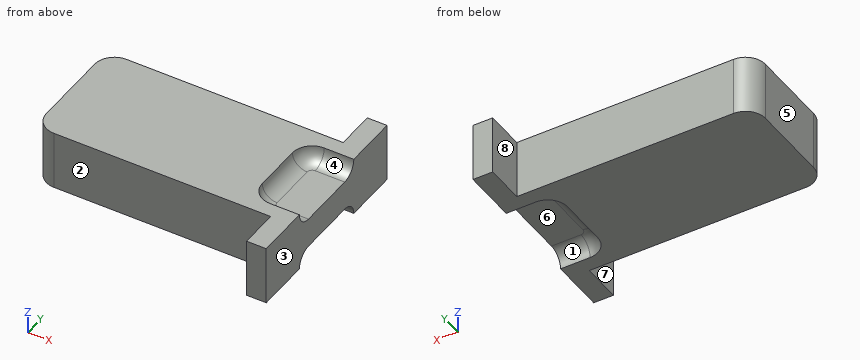
from build123d import *

# Parameters (mm, degrees)
F1_DEPTH = 9.525
F2_R     = 6.35
F4_DEPTH = 4.7625
F5_R     = 4.76249
F7_DEPTH = 4.7625
F8_R     = 4.76249


# Not quite as in the source:
# - a fillet or chamfer is up to 0.001 mm smaller than in the source, because OpenCascade refuses the exact size


with BuildPart() as f1:
    # F0 (on Top) → F1 (new body, symmetric)
    with BuildSketch(Plane.XY):
        Polygon((-82.55, 19.05), (-82.55, -19.05), (-6.35, -19.05), (-6.35, -31.75), (0, -31.75), (0, 31.75), (-6.35, 31.75), (-6.35, 19.05), align=None)
    extrude(amount=F1_DEPTH, both=True)

    # F2
    f2_edges = [f1.edges().sort_by_distance(p)[0] for p in [
        (-82.55, -19.05, 0),
        (-82.55, 19.05, 0),
    ]]
    fillet(f2_edges, radius=F2_R)

    # F3 (on face) → F4 (cut)
    with BuildSketch(Plane.XY.offset(9.525)):
        with BuildLine():
            Line((0, -14.2875), (0, 14.2875))
            Line((0, 14.2875), (-9.525, 14.2875))
            ThreePointArc((-9.525, 14.2875), (-14.0151280605, 12.4276280605), (-15.875, 7.9375))
            Line((-15.875, 7.9375), (-15.875, -7.9375))
            ThreePointArc((-15.875, -7.9375), (-14.0151280605, -12.4276280605), (-9.525, -14.2875))
            Line((-9.525, -14.2875), (0, -14.2875))
        make_face()
    extrude(amount=-F4_DEPTH, mode=Mode.SUBTRACT)

    # F5 (radius 4.7625 in the source; OpenCascade refuses exactly that, so slightly less here)
    f5_edges = [f1.edges().sort_by_distance(p)[0] for p in [
        (-4.7625, 14.2875, 4.7625),
        (-14.015128, 12.427628, 4.7625),
    ]]
    fillet(f5_edges, radius=F5_R)

    # F6 (on face) → F7 (cut)
    with BuildSketch(Plane(origin=(0, 0, -9.525), x_dir=(1, 0, 0), z_dir=(0, 0, -1))):
        with BuildLine():
            Line((0, -14.2875), (0, 14.2875))
            Line((0, 14.2875), (-9.525, 14.2875))
            ThreePointArc((-9.525, 14.2875), (-14.0151280605, 12.4276280605), (-15.875, 7.9375))
            Line((-15.875, 7.9375), (-15.875, -7.9375))
            ThreePointArc((-15.875, -7.9375), (-14.0151280605, -12.4276280605), (-9.525, -14.2875))
            Line((-9.525, -14.2875), (0, -14.2875))
        make_face()
    extrude(amount=-F7_DEPTH, mode=Mode.SUBTRACT)

    # F8 (radius 4.7625 in the source; OpenCascade refuses exactly that, so slightly less here)
    f8_edges = [f1.edges().sort_by_distance(p)[0] for p in [
        (-4.7625, -14.2875, -4.7625),
        (-14.015128, -12.427628, -4.7625),
    ]]
    fillet(f8_edges, radius=F8_R)


solid = f1.part
For this review, take the finished solid that the model builds, in its own axes (mm). Face numbers are marked on the shaded views. A direction names the side the tool comes from. Coordinates: 2 decimals unless noted, no trailing zeros. Loops run counter-clockwise (first coordinate to the right, second up) from the corner with the lowest first, then second, coordinate; pieces in that order, holes last. Notation, with made-up numbers: (60.5, 24.5) - (74.5, 24.5) arc R23 cw to (74.5, 61.5) - close; hole circle Ø9 at (44, 5). An arc over 180 degrees is marked (long way). Use a Markdown table: item, result. Add a question column.
Item 1: We need section D-D (y = -28). Give the boundary of the cut face in (x, z) (3 decimals), and give its area (3 significant figures).
Item 2: For line 1 (X direction, y = 28, z = -6); line 2 (Y direction, x = -27, z = 4), list the stretches that pass through material, from the lowest coordinate up.
Item 3: Insertion check: pin 1 Ø1.5 at (x, z) = (-32.5, 2.5) entering from -Y; pin 2 Ø5.5 at (x, y) = (-8.5, 0.5) entering from -Z; pin 3 Ø1.5 at (x, y) = (-11.5, 8.5) entering from +Z. Each pin has a flat end and moves straight along its axis. Give the tip position at first contact, or say it passes through.
Item 4: We need section B-B (z = -2.25). Give the boundary of the cut face in (x, y), and give its area (3 significant figures).
Item 5: Tool access review of the marked faces 4, 5, 6, 7 and 8: name each direction out of +Z, -Z, +X, -X, +Y, -Y from which nothing blocks a thin tool from reaching the whole face with its end or side.
Item 6: Mouldability with a two-part tool opening along Y and no side actions: class the marked faces 1, 2 and 3 as pulls with the +Y half, pulls with the -Y half, needs draft (parallel to the pull), parting line crosses it, or undercut.
Item 7: We need section C-C (x = -70). Give the boundary of the cut face in (y, z) (3 decimals).
Results list:
| question | item | result |
|---|---|---|
| 1 | outline | (-6.35, -9.525) - (0, -9.525) - (0, 9.525) - (-6.35, 9.525) - close |
| 1 | area | 121 mm^2 |
| 2 | line 1 | x = -6.35 to 0 |
| 2 | line 2 | y = -19.05 to 19.05 |
| 3 | pin 1 | stops at y = -19.05 |
| 3 | pin 2 | stops at z = -4.76 |
| 3 | pin 3 | stops at z = 4.92 |
| 4 | outline | (-82.55, -12.7) arc R6.35 ccw to (-76.2, -19.05) - (-6.35, -19.05) - (-6.35, -31.75) - (0, -31.75) - (0, 31.75) - (-6.35, 31.75) - (-6.35, 19.05) - (-76.2, 19.05) arc R6.35 ccw to (-82.55, 12.7) - close |
| 4 | area | 3,290 mm^2 |
| 5 | face 4 | +Z, +X |
| 5 | face 5 | +Z, -Z, -X, +Y, -Y |
| 5 | face 6 | -Z, +X |
| 5 | face 7 | +Z, -Z, -X, -Y |
| 5 | face 8 | +Z, -Z, -X, +Y |
| 6 | face 1 | undercut |
| 6 | face 2 | pulls with the -Y half |
| 6 | face 3 | needs draft |
| 7 | outline | (-19.05, -9.525) - (19.05, -9.525) - (19.05, 9.525) - (-19.05, 9.525) - close |
